Autodesk Inventor part; units mm, degrees
ref_plane "YZ Plane" through (0, 0, 0) normal (1, 0, 0) x (0, 1, 0)
ref_plane "XZ Plane" through (0, 0, 0) normal (0, 1, 0) x (-1, 0, 0)
ref_plane "XY Plane" through (0, 0, 0) normal (0, 0, 1) x (1, 0, 0)
sketch "Sketch1" plane through (0, 0, 0) normal (0, 0, 1) x (1, 0, 0)
  line L0 (0, 0) -> (200, 0)
  line L1 (200, 0) -> (200, 85)
  line L2 (200, 85) -> (0, 85)
  line L3 (0, 85) -> (0, 0)
  dimension "d0" = 200
  dimension "d1" = 85
extrude "Extrusion1" add sketch "Sketch1" along normal blind 19
sketch "Sketch2" plane through (200, 0, 0) normal (1, 0, 0) x (0, 0, -1)
  line L0 (0, 0) -> (-19, 0)
  line L1 (0, 85) -> (-19, 85)
  line L2 (-19, 0) -> (-19, 14.605)
  line L3 (-19, 0) -> (-19, 85)
  arc A0 (-19, 14.605) -> (-19, 85) centre (-79.4534, 49.8025) ccw
  dimension "d9" = 14.605
extrude "Extrusion2" cut sketch "Sketch2" against normal through all
sketch "Sketch9" plane through (0, 0, 19) normal (0, 0, 1) x (1, 0, 0)
  line L0 (200, 14.605) -> (0, 14.605)
  line L1 (0, 14.605) -> (0, 85)
  arc A0 (40.2378, 14.605) -> (0, 45.6428) centre (-0.879, 2.9021) ccw
  line L2 (0, 45.6428) -> (0, 14.605)
  line L3 (49.8468, 14.605) -> (0, 14.605)
  arc A1 (34.584, 26.7752) -> (49.8468, 14.605) centre (58.9671, 41.6987) ccw
  point P0 (0, 0)
  point P1 (38.109, 20.4373)
extrude "Extrusion6" add sketch "Sketch9" against normal blind 12.7 contours L0 A0 A1 | L0 L1 A0 A1
fillet "Fillet4" radius 3.175 2 edges at (19.5949, 40.4303, 19) (41.1444, 19.347, 19)
sketch "Sketch10" plane through (0, 0, 19) normal (0, 0, 1) x (1, 0, 0)
  line L0 (21.6079, 10.4672) -> (13.9879, 6.0678)
  line L1 (13.9879, 6.0678) -> (6.3679, 10.4672)
  line L2 (6.3679, 29.8109) -> (13.9879, 34.2103)
  line L3 (13.9879, 34.2103) -> (21.6079, 29.8109)
  line L4 (6.3679, 29.8109) -> (6.3679, 10.4672)
  line L5 (21.6079, 29.8109) -> (21.6079, 10.4672)
  point P0 (0, 0)
  point P1 (13.9879, 20.1391)
  dimension "d24" = 28.1426
  dimension "d29" = 15.24
  dimension "d30" = 4.3994
extrude "Extrusion7" cut sketch "Sketch10" against normal blind 3
fillet "Fillet5" radius 3.302 6 edges at (13.9879, 34.2103, 17.5) (21.6079, 29.8109, 17.5) (6.3679, 29.8109, 17.5) (6.3679, 10.4672, 17.5) (13.9879, 6.0678, 17.5) (21.6079, 10.4672, 17.5)
sketch "Sketch11" plane through (0, 0, 16) normal (0, 0, 1) x (1, 0, 0)
  arc A0 (19.9569, 9.514) -> (21.6079, 12.3736) centre (18.3059, 12.3736) ccw
  line L0 (21.6079, 27.9045) -> (21.6079, 12.3736)
  arc A1 (21.6079, 27.9045) -> (19.9569, 30.7641) centre (18.3059, 27.9045) ccw
  line L1 (15.6389, 33.2571) -> (19.9569, 30.7641)
  arc A2 (15.6389, 33.2571) -> (12.3369, 33.2571) centre (13.9879, 30.3975) ccw
  line L2 (8.0189, 30.7641) -> (12.3369, 33.2571)
  arc A3 (8.0189, 30.7641) -> (6.3679, 27.9045) centre (9.6699, 27.9045) ccw
  line L3 (6.3679, 12.3736) -> (6.3679, 27.9045)
  arc A4 (6.3679, 12.3736) -> (8.0189, 9.514) centre (9.6699, 12.3736) ccw
  line L4 (12.3369, 7.021) -> (8.0189, 9.514)
  arc A5 (12.3369, 7.021) -> (15.6389, 7.021) centre (13.9879, 9.8806) ccw
  line L5 (19.9569, 9.514) -> (15.6389, 7.021)
  point P0 (0, 0)
properties part number "prototype #1"
Source: CAD feature listing. Evaluate the final solid. Frame: model axes, mm. A direction names the side the tool comes from. Give positions to 0.01 mm unless a question says otherwise; leave off trailing zeros. Loops run counter-clockwise (first coordinate to the right, second up) from the corner with the lowest first, then second, coordinate; pieces in that order, holes last. Notation, with made-up numbers: (-9.75, 39.25) -> (21.25, 39.25) arc R9 cw to (21.25, 53.25) -> close; hole circle Ø11 at (-17.75, -8.75). An arc over 180 degrees is marked (long way). Put each result on its own line as item: value. Start each with the question number.
1) Material intervals for probe 1 along Z at (x, y) = (163, 53.5); probe 2 along X at (y, z) = (28, 16.75); probe 3 along X at (y, z) = (18, 18.25), sorted ascending.
2) Reachability of faces 1 (the face through (19.85, 40.29, 12.77)), 2 (the face through (14, 20, 16)), 3 (the face through (99, 12, 19)) from +Z, -Z, +X, -X, +Y, -Y: full face, straight path, thin tool, end or side. Return the list, or none.
3) Contact query for flat-ended pins moving along their axis: P1, Ø5, axis at x = 21, y = 76, coming from the +Z side; P2, Ø1.5, axis at y = 20.5, z = 17, coming from the +X side; P3, Ø4, axis at x = 142, y = 17.5, coming from the +Z side. Output: stop coordinate, or through.
4) Cut plane A-A (x = 157). Return loops of the section in (y, z) (1 decimal), then the cut area to 3 significant figures.
5) Cut plane C-C (y = 51). Return loops of the section in (x, z).
6) Cut plane B-B (y = 66.5). Return loops of the section in (x, z).
Results are:
1. probe 1: z = 0 to 9.6
1. probe 2: x = 0 to 6.37, 21.61 to 33.56
1. probe 3: x = 0 to 6.37, 21.61 to 41.04
2. face 1: +Z, +X
2. face 2: +Z
2. face 3: +Z, +X, -X, +Y, -Y
3. P1: stops at z = 15.66
3. P2: stops at x = 40.39
3. P3: stops at z = 18.49
4. outline: (0, 0) -> (85, 0) -> (85, 19) arc R70 cw to (14.6, 19) -> (0, 19) -> close
4. area: 1,160 mm2
5. outline: (0, 0) -> (200, 0) -> (200, 9.51) -> (0, 9.51) -> close
6. outline: (0, 0) -> (200, 0) -> (200, 11.52) -> (0, 11.52) -> close
